Geometry check sheet. Reference: the model listing, model coordinates, mm. Face numbers are marked on the shaded views. A direction names the side the tool comes from. Give positions to 0.01 mm unless a question says otherwise; leave off trailing zeros. Loops run counter-clockwise (first coordinate to the right, second up) from the corner with the lowest first, then second, coordinate; pieces in that order, holes last. Notation, with made-up numbers: (58, 47.5) - (92, 47.5) arc R7 cw to (92, 51.5) - close; hole circle Ø11 at (76, 9.5). An arc over 180 degrees is marked (long way). Use a Markdown table: item, result. Add a question column.
1. Cross-section at A-A on z = 6.42. Count the separate pieces of the cut face and the enclosed holes in it, and give its area (3 significant figures).
2. Material ranges on L1, parallel to X at y = -10.9, z = 6.42; L2, parallel to Z at x = 19.54, y = -9.45; L3, parallel to X at y = -7.5, z = 9.25, recorded low to high.
3. Draft check along Z on the marked faces 4, 5, 6 and 7. Enter one of: pulls with the +Z half, pulls with the -Z half, needs draft (parallel to the pull), parting line crosses it, or undercut.
4. Depth check by flat-ended pin: P1, Ø5, axis at y = -1.5, z = 3, coming from the -X side; P2, Ø5.5, axis at x = 18, y = -6.5, coming from the -Z side; P3, Ø4, axis at y = -6, z = 4, coming from the +X side; P4, Ø3, axis at x = 19.54, z = 6.42, coming from the +Y side. Enter the tip coordinate at first touch or a pass-through.
5. Set-up check for the marked faces 1, 2 and 3: record each of +Z, -Z, +X, -X, +Y, -Y from which the full face is reachable in a straight line by a thin tool's end or side.
6. Cross-section at D-D on x = 18.5. Enter the section's corners in (y, z), and give its area (3 significant figures).
7. Cross-section at C-C on y = -4. Enter the section's corners in (x, z).
8. Cross-section at B-B on y = -11. Enter the section's corners in (x, z) (1 decimal).
from build123d import *

# Parameters (mm, degrees)
BOSS_EXTRUDE1_DEPTH     = 11.5
FILLET1_R               = 2
BOSS_EXTRUDE2_DEPTH     = 5.08
FILLET2_R               = 2
FILLET3_R               = 2
SKETCH3_R               = 1.5875
CUT_EXTRUDE1_DEPTH      = 30.958731615
CUT_EXTRUDE3_DEPTH      = 2
CUT_EXTRUDE3_DEPTH_BACK = 2.54
CUT_EXTRUDE3_START      = 5.08


with BuildPart() as part:
    # Sketch1 → Boss-Extrude1 (new body)
    with BuildSketch(Plane.XY):
        Polygon((1.5, -11.5), (1.5, -1.5), (13.5, -1.5), (13.5, -11.5), (15, -11.5), (15, 0), (0, 0), (0, -11.5), align=None)
    extrude(amount=BOSS_EXTRUDE1_DEPTH)

    # Fillet1
    fillet1_edges = [part.edges().sort_by_distance(p)[0] for p in [
        (13.5, -1.5, 5.75),
        (1.5, -1.5, 5.75),
    ]]
    fillet(fillet1_edges, radius=FILLET1_R)

    # Sketch2 → Boss-Extrude2 (add)
    with BuildSketch(Plane(origin=(0, -11.5, 0), x_dir=(1, 0, 0), z_dir=(0, 1, 0))):
        with BuildLine():
            Line((15, -1.34), (15, -11.5))
            Line((15, -11.5), (20.08, -11.5))
            ThreePointArc((20.08, -11.5), (25.16, -6.42), (20.08, -1.34))
            Line((20.08, -1.34), (15, -1.34))
        make_face()
        with BuildLine():
            Line((0, -1.34), (-5.08, -1.34))
            ThreePointArc((-5.08, -1.34), (-10.16, -6.42), (-5.08, -11.5))
            Line((-5.08, -11.5), (0, -11.5))
            Line((0, -11.5), (0, -1.34))
        make_face()
    extrude(amount=BOSS_EXTRUDE2_DEPTH)

    # Fillet2
    fillet2_edges = [part.edges().sort_by_distance(p)[0] for p in [
        (15, -6.42, 6.42),
        (0, -6.42, 6.42),
    ]]
    fillet(fillet2_edges, radius=FILLET2_R)

    # Fillet3
    fillet3_edges = [part.edges().sort_by_distance(p)[0] for p in [
        (15, 0, 5.75),
        (0, 0, 5.75),
    ]]
    fillet(fillet3_edges, radius=FILLET3_R)

    # Sketch3 → Cut-Extrude1 (cut, through all)
    with BuildSketch(Plane(origin=(0, -11.5, 0), x_dir=(1, 0, 0), z_dir=(0, 1, 0))):
        with Locations(Location((19.54, -6.42, 0), (0, 0, 270))):
            Circle(SKETCH3_R)
        with Locations(Location((-4.54, -6.42, 0), (0, 0, 90))):
            Circle(SKETCH3_R)
    extrude(amount=CUT_EXTRUDE1_DEPTH, mode=Mode.SUBTRACT)

    # Sketch6 → Cut-Extrude3 (cut, two sides: drawn at the far end of the back side and taken through both)
    with BuildSketch(Plane(origin=(0, -11.5, 0), x_dir=(1, 0, 0), z_dir=(0, 1, 0)).offset(CUT_EXTRUDE3_START - CUT_EXTRUDE3_DEPTH_BACK)):
        Polygon((-1.365, -4.586912895), (-4.54, -2.753825791), (-7.715, -4.586912895), (-7.715, -8.253087105), (-4.54, -10.086174209), (-1.365, -8.253087105), align=None)
        Polygon((22.715, -8.253087105), (22.715, -4.586912895), (19.54, -2.753825791), (16.365, -4.586912895), (16.365, -8.253087105), (19.54, -10.086174209), align=None)
    extrude(amount=CUT_EXTRUDE3_DEPTH + CUT_EXTRUDE3_DEPTH_BACK, mode=Mode.SUBTRACT)


solid = part.part
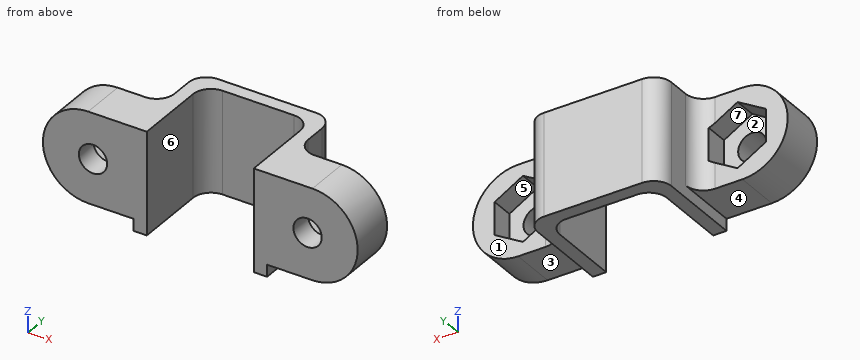
Values found:
| question | item | result |
|---|---|---|
| 1 | separate pieces | 3 |
| 1 | enclosed holes | 0 |
| 1 | area | 109 mm2 |
| 2 | L1 | x = -10.16 to -6.13, -2.95 to 1.5, 13.5 to 17.95, 21.13 to 25.16 |
| 2 | L2 | z = 1.34 to 4.83, 8.01 to 11.5 |
| 2 | L3 | x = -9.3 to -5.99, -3.09 to 1.5, 13.5 to 18.09, 20.99 to 24.3 |
| 3 | face 4 | pulls with the -Z half |
| 3 | face 5 | undercut |
| 3 | face 6 | needs draft |
| 3 | face 7 | undercut |
| 4 | P1 | stops at x = 0 |
| 4 | P2 | stops at z = 1.34 |
| 4 | P3 | stops at x = 25.14 |
| 4 | P4 | passes through |
| 5 | face 1 | +Z, -Z, +X, +Y |
| 5 | face 2 | +Y |
| 5 | face 3 | -Z, +X, +Y, -Y |
| 6 | outline | (-11.5, 1.34) - (-6.42, 1.34) - (-6.42, 3.35) - (-8.96, 3.35) - (-8.96, 5.22) - (-11.5, 5.22) - close; (-11.5, 7.62) - (-8.96, 7.62) - (-8.96, 9.49) - (-6.42, 9.49) - (-6.42, 11.5) - (-11.5, 11.5) - close |
| 6 | area | 29.9 mm2 |
| 7 | outline | (0, 0) - (1.5, 0) - (1.5, 11.5) - (0, 11.5) - close; (13.5, 0) - (15, 0) - (15, 11.5) - (13.5, 11.5) - close |
| 8 | outline | (-5.1, 1.3) - (0, 1.3) - (0, 0) - (1.5, 0) - (1.5, 11.5) - (-5.1, 11.5) arc R5.1 ccw to start; (13.5, 0) - (15, 0) - (15, 1.3) - (20.1, 1.3) arc R5.1 ccw to (20.1, 11.5) - (13.5, 11.5) - close; hole circle Ø3.2 at (-4.5, 6.4); hole circle Ø3.2 at (19.5, 6.4) |
